Verification items for the finished model (mm, model axes). A direction names the side the tool comes from. Coordinates: 2 decimals unless noted, no trailing zeros. Loops run counter-clockwise (first coordinate to the right, second up) from the corner with the lowest first, then second, coordinate; pieces in that order, holes last.
Q1. Go/stop test with flat-tipped pins: P1, Ø1, axis at x = 1.5, z = -9.5, coming from the +Y side; P2, Ø1.9, axis at x = 1.5, y = 11.5, coming from the -Z side; P3, Ø1.5, axis at x = 0.5, y = 150, coming from the -Z side; P4, Ø9, axis at y = 270, z = -20, coming from the +X side. Record where each tip stops, or that it passes through.
Q2. Material ranges on probe 1 along Y at (x, z) = (1.5, -20) (3 decimals); probe 2 along Z at (x, y) = (-0.25, 11); probe 3 along Z at (x, y) = (1.5, 0) (3 decimals), recorded low to high.
Q3. Access from +Z, -Z, +X, -X, +Y, -Y to the whole of each face (thin tool, end or side, straight path). Record for faces 5 (the face through (3.175, 156, -17)), 6 (the face through (0.044, 263.476, -28.301)), 7 (the face through (-0.044, 254.788, -30.349)), 8 (the face through (0, 67, -8)), 9 (the face through (0, -8, 0)).
Q4. Sectioned sample at A-A (z = -20). Enter the section's corners in (x, y) (3 decimals), then the cut area to 3 significant figures.
Q5. Sectioned sample at C-C (y = 122). Enter the section's corners in (x, z) (3 decimals).
Q6. Mould release check, pull along Y, two halves, no side actions. Record for faces 1 (the face through (0.04, 266.01, -29.91)), 2 (the face through (-3.175, 156, -17)), 3 (the face through (-0.04, 141.85, 7.24)), 4 (the face through (-0.04, 246.87, -62.95)): +Y half, -Y half, draft (parallel to the pull), parting line (faces both ways), or undercut.
Q7. Sectioned sample at D-D (y = 181.5). Enter the section's corners in (x, z) (3 decimals), then the cut area to 3 significant figures.
Q8. Sectioned sample at B-B (x = 0.75). Count the separate pieces of the cut face and the enclosed holes in it, then the cut area to 3 significant figures.
Autodesk Inventor part; units mm, degrees
ref_plane "YZ Plane" through (0, 0, 0) normal (1, 0, 0) x (0, 1, 0)
ref_plane "XZ Plane" through (0, 0, 0) normal (0, 1, 0) x (-1, 0, 0)
ref_plane "XY Plane" through (0, 0, 0) normal (0, 0, 1) x (1, 0, 0)
sketch "Sketch1" plane through (0, 0, 0) normal (1, 0, 0) x (0, 1, 0)
  line L0 (-10, -10) -> (10, -10) construction
  line L1 (10, -10) -> (10, 10) construction
  line L2 (10, 10) -> (-10, 10) construction
  line L3 (-10, 10) -> (-10, -10) construction
  line L4 (-10, -10) -> (10, 10) construction
  line L5 (10, -10) -> (-10, 10) construction
  line L6 (0, 0) -> (135.9808, 0)
  line L7 (253.6603, -48.3013) -> (270, -20)
  line L8 (114.9075, -11.5) -> (119.815, -20) construction
  line L9 (119.815, -20) -> (114.9075, -28.5) construction
  line L10 (114.9075, -28.5) -> (105.0925, -28.5) construction
  line L11 (105.0925, -28.5) -> (100.185, -20) construction
  line L12 (100.185, -20) -> (105.0925, -11.5) construction
  line L13 (105.0925, -11.5) -> (114.9075, -11.5) construction
  line L14 (143.4808, -2.0096) -> (233.1699, -53.7917)
  arc A0 (233.1699, -53.7917) -> (253.6603, -48.3013) centre (240.6699, -40.8013) ccw
  arc A1 (143.4808, -2.0096) -> (135.9808, 0) centre (135.9808, -15) ccw
  point P0 (140, 0)
  point P1 (246.1603, -61.2917)
  point P2 (110, -20)
  dimension "d0" = 270
  dimension "d4" = 20
  dimension "d5" = 20
  dimension "d60" = 20
  dimension "d65" = 17
  dimension "d66" = 160
  dimension "d68" = 11.5
  dimension "d82" = 150
  dimension "d83" = 140
  dimension "d84" = 15
  dimension "d93" = 15
surface extrude "ExtrusionSrf1" sketch "Sketch1" along normal mid plane 6.35 shown no curves L6 A1 L14 A0 L7
thicken "Thicken1" operation new thickness 16 both sides yes extend neighbours no toward (0, 0, 1) faces at (-1.0583, 45.3269, 0) (1.0583, 139.44, -0.4043) (1.0583, 173.3771, -19.2703) (1.0583, 244.0077, -55.4252) (-1.0583, 259.1068, -38.8675)
sketch "Sketch4" plane through (3.175, 0, 8) normal (1, 0, 0) x (0, 0, -1)
  line L0 (60.3013, 260.5885) -> (32, 276.9282)
  line L1 (32, 276.9282) -> (24, 263.0718)
  line L2 (52.3013, 246.7321) -> (24, 263.0718)
  arc A0 (54.8634, 237.1699) -> (52.3013, 246.7321) centre (48.8013, 240.6699) ccw
  line L3 (3.0814, 147.4808) -> (54.8634, 237.1699)
  line L4 (0, 0) -> (0, 135.9808)
  line L5 (16, 0) -> (0, 0)
  line L6 (16, 0) -> (16, 135.9808)
  line L7 (16.9378, 139.4808) -> (68.7199, 229.1699)
  arc A1 (68.7199, 229.1699) -> (60.3013, 260.5885) centre (48.8013, 240.6699) ccw
  line L8 (16, 0) -> (0, 0)
  circle A2 centre (8, 0) radius 8
  circle A3 centre (28, 270) radius 8
  arc A4 (3.0814, 147.4808) -> (0, 135.9808) centre (23, 135.9808) ccw
  arc A5 (16.9378, 139.4808) -> (16, 135.9808) centre (23, 135.9808) ccw
extrude "Extrusion2" add sketch "Sketch4" against normal up to surface (6.35 mm away) contours L1 A3 | A2 L5 | L5 A2 picked at (25.5467, 271.0452)
hole "Hole4" at (3.175, 0, 0) at (3.175, 270, -20) direction (-1, 0, 0) diameter 11.05 end through all
sketch "Sketch5" plane through (3.175, 0, 0) normal (1, 0, 0) x (0, 0, -1)
  line L0 (-8, 0) -> (-8, 135.9808)
  arc A0 (-8, 0) -> (8, 0) centre (0, 0) ccw
  line L1 (8, 0) -> (8, 135.9808)
  line L2 (8.9378, 139.4808) -> (60.7199, 229.1699)
  arc A1 (60.7199, 229.1699) -> (52.3013, 260.5885) centre (40.8013, 240.6699) ccw
  line L3 (52.3013, 260.5885) -> (24, 276.9282)
  arc A2 (24, 276.9282) -> (16, 263.0718) centre (20, 270) ccw
  line L4 (44.3013, 246.7321) -> (16, 263.0718)
  arc A3 (46.8634, 237.1699) -> (44.3013, 246.7321) centre (40.8013, 240.6699) ccw
  line L5 (-4.9186, 147.4808) -> (46.8634, 237.1699)
  circle A4 centre (0, 0) radius 5.525
  circle A5 centre (20, 270) radius 5.525
  line L6 (20, 270) -> (32.9904, 262.5) construction
  line L7 (19.25, 268.701) -> (32.2404, 261.201)
  line L8 (33.7404, 263.799) -> (20.75, 271.299)
  arc A6 (20.75, 271.299) -> (19.25, 268.701) centre (20, 270) ccw
  arc A7 (32.2404, 261.201) -> (33.7404, 263.799) centre (32.9904, 262.5) ccw
  line L9 (0, 0) -> (0, 15) construction
  line L10 (1.5, 0) -> (1.5, 15)
  line L11 (-1.5, 15) -> (-1.5, 0)
  arc A8 (-1.5, 0) -> (1.5, 0) centre (0, 0) ccw
  arc A9 (1.5, 15) -> (-1.5, 15) centre (0, 15) ccw
  arc A10 (8.9378, 139.4808) -> (8, 135.9808) centre (15, 135.9808) ccw
  arc A11 (-4.9186, 147.4808) -> (-8, 135.9808) centre (15, 135.9808) ccw
  point P0 (0, 0)
  point P1 (26.4952, 266.25)
  point P2 (0, 7.5)
  point P3 (-1.5, 5.3175)
  point P4 (1.5, 5.3175)
  point P5 (25.3551, 268.6403)
  point P6 (23.8551, 266.0422)
  dimension "d86" = 3
  dimension "d87" = 15
extrude "Extrusion3" cut sketch "Sketch5" against normal through all contours A4 L11 A9 L10 | A5 L8 A7 L7
fillet "Fillet4" radius 1 4 edges at (0, 266.0422, -23.8551) (0, 268.6403, -25.3551) (0, 5.3175, 1.5) (0, 5.3175, -1.5)
properties part number "Door Upper Parallel Bar"
Geometry check:
1. P1: stops at y = 173.32
1. P2: stops at z = -8
1. P3: stops at z = -15.44
1. P4: passes through
2. probe 1: y = 158.641 to 190.641, 260.762 to 264.475, 275.525 to 278
2. probe 2: z = -8 to -1.5, 1.5 to 8
2. probe 3: z = -8 to -5.525, 5.525 to 8
3. face 5: +Z, -Z, +X, +Y, -Y
3. face 6: +X, -X
3. face 7: +Z, +X, -X
3. face 8: -Z, +X, -X, -Y
3. face 9: +X, -X, -Y
4. outline: (-3.175, 158.641) - (3.175, 158.641) - (3.175, 190.641) - (-3.175, 190.641) - close; (-3.175, 260.762) - (3.175, 260.762) - (3.175, 264.475) - (-3.175, 264.475) - close; (-3.175, 275.525) - (3.175, 275.525) - (3.175, 278) - (-3.175, 278) - close
4. area: 242 mm2
5. outline: (-3.175, -8) - (3.175, -8) - (3.175, 8) - (-3.175, 8) - close
6. face 1: undercut
6. face 2: draft
6. face 3: +Y half
6. face 4: parting line
7. outline: (-3.175, -33.198) - (3.175, -33.198) - (3.175, -14.722) - (-3.175, -14.722) - close
7. area: 117 mm2
8. separate pieces: 1
8. enclosed holes: 2
8. area: 4,800 mm2
